Part model, mm, in its own coordinate system. Face numbers are marked on the shaded views. A direction names the side the tool comes from. Round coordinates to 2 decimals unless told otherwise and drop trailing zeros. Order: outer loops, then holes, each group sorted by start corner. A loop starts at its lowest first (then second) coordinate and runs counter-clockwise, first axis right, second up. Notation, with made-up numbers: (-12, 86) - (45, 86) arc R23 cw to (45, 100) - close; hole circle Ø5 at (0.25, 25.5). An arc over 180 degrees is marked (long way). Return JSON: item names as keys, results as strings. Group by question number.
Item 1: Drop flat-ended pins along their axis: pin 1 (21 mm diameter, centred on x = 0, z = -81, fed in from -Y); pin 2 (1 mm diameter, centred on x = -66, z = 123, fed in from -Y); pin 3 (6 mm diameter, centred on x = 59, z = -204.5, fed in from +Y). Give the stop position or say it passes through.
Item 2: Two-plate mould, pull along X, no slides. Class the marked faces 1, 2, 3 and 4: released by +X, released by -X, zero draft, split by the parting line, or undercut.
Item 3: Tool access for the marked faces 5, 6, 7 and 8: list every direction of +Z, -Z, +X, -X, +Y, -Y with a clear straight run to the whole face (end or side of a thin tool).
Item 4: Saw through at A-A on y = 80. List the corners of the cut face in (x, z), and give its area (3 significant figures).
Item 5: Probe probe 1 along Z at (x, y) = (0, -5); probe 2 along X at (y, z) = (-5.25, 0). List the from-to ranges inside material, lowest first.
```python
from build123d import *

# Parameters (mm, degrees)
THICKEN1_T1            = 8
CUT_EXTRUDE1_DEPTH     = 485.367654355
CIRPATTERN1_COUNT      = 6
F_16_0MM_DOWEL_HOLE2_D = 16
CIRPATTERN2_COUNT      = 8


with BuildPart() as body_1:
    # Surface-Revolve1: a surface, the sketch's curves turned about an axis
    with BuildLine(Plane.XY, mode=Mode.PRIVATE) as surface_revolve1_1_path:
        Line((53, 0), (115, 0))
        ThreePointArc((115, 0), (143.012028142, -16.093774461), (168.057295138, 4.312545592))
        Line((168.057295138, 4.312545592), (198.057295138, 4.312545592))
        ThreePointArc((198.057295138, 4.312545592), (219.254065707, 10.390621746), (234.00905699, 26.77769972))
        Line((234.00905699, 26.77769972), (269.721959046, 100))
        Line((269.721959046, 100), (332.5, 100))
    surface_revolve1_1 = Shell.revolve(surface_revolve1_1_path.wire(), 360, Axis((0, 0, 0), (0, 1, 0)))
    add(Solid.thicken(surface_revolve1_1, THICKEN1_T1))

    # Sketch2 → Cut-Extrude1 (cut, through all)
    with BuildSketch(Plane.XZ.offset(-92)):
        with BuildLine():
            ThreePointArc((-278.018608961, 182.378461095), (-137.025263873, 238.108499582), (-18, 332.012424466))
            ThreePointArc((-18, 332.012424466), (-165.844309403, 288.187291598), (-278.018608961, 182.378461095))
        make_face()
        with BuildLine():
            ThreePointArc((0, 320), (-10, 310), (0, 300))
            Line((0, 300), (0, 320))
        make_face()
        with BuildLine():
            Line((0, 320), (0, 300))
            ThreePointArc((0, 300), (7.071067812, 302.928932188), (10, 310))
            ThreePointArc((10, 310), (7.071067812, 317.071067812), (0, 320))
        make_face()
    cut_extrude1 = extrude(amount=-CUT_EXTRUDE1_DEPTH, mode=Mode.SUBTRACT)

    # CirPattern1: Cut-Extrude1 ×6 about axis
    cirpattern1_axis = Axis((0, 0, 0), (0, 1, 0))
    for i in range(1, CIRPATTERN1_COUNT):
        add(cut_extrude1.rotate(cirpattern1_axis, i * 360 / CIRPATTERN1_COUNT), mode=Mode.SUBTRACT)

    # Ø16.0mm Dowel Hole2 (through all)
    with Locations(Plane(origin=(0, 0, 0), x_dir=(1, 0, 0), z_dir=(0, 1, 0))):
        with Locations((0, 81)):
            f_16_0mm_dowel_hole2 = Hole(F_16_0MM_DOWEL_HOLE2_D / 2)

    # CirPattern2: Ø16.0mm Dowel Hole2 ×8 about axis
    cirpattern2_axis = Axis((0, 0, 0), (0, 1, 0))
    for i in range(1, CIRPATTERN2_COUNT):
        add(f_16_0mm_dowel_hole2.rotate(cirpattern2_axis, i * 360 / CIRPATTERN2_COUNT), mode=Mode.SUBTRACT)


solid = body_1.part
```
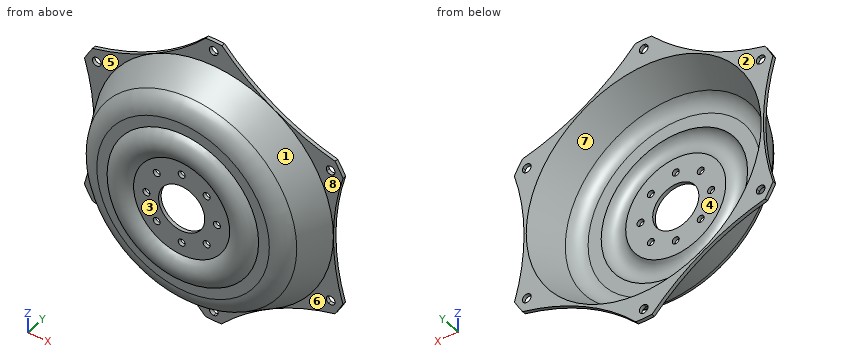
Filled in:
{
 "1": {"pin 1": "stops at y = -8", "pin 2": "stops at y = -24.18", "pin 3": "stops at y = 8.48"},
 "2": {"face 1": "split by the parting line", "face 2": "zero draft", "face 3": "undercut", "face 4": "undercut"},
 "3": {"face 5": "+Z, -X, -Y", "face 6": "-Z, +X, -Y", "face 7": "+Y", "face 8": "+Z, +X, -Y"},
 "4": {"outline": "circle Ø537.74 at (0, 0); hole circle Ø519.93 at (0, 0)", "area": "14,800 mm^2"},
 "5": {"probe 1": "z = -172.84 to -163.34, -118.06 to -89, -73 to -53, 53 to 73, 89 to 118.06, 163.34 to 172.84", "probe 2": "x = -172.7 to -163.15, -118.26 to -89, -73 to -53, 53 to 73, 89 to 118.26, 163.15 to 172.7"}
}
